Source: CAD feature listing. Evaluate the final solid. Frame: model axes, mm. Face numbers are marked on the shaded views. A direction names the side the tool comes from. Give positions to 0.01 mm unless a question says otherwise; leave off trailing zeros. Order: outer loops, then holes, each group sorted by start corner. A loop starts at its lowest first (then second) coordinate and runs counter-clockwise, first axis right, second up.
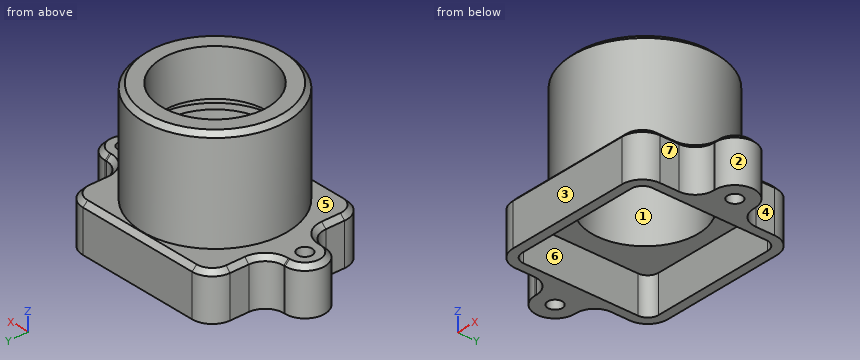
Autodesk Inventor part; units mm, degrees
ref_plane "YZ Plane" through (0, 0, 0) normal (1, 0, 0) x (0, 1, 0)
ref_plane "XZ Plane" through (0, 0, 0) normal (0, 1, 0) x (-1, 0, 0)
ref_plane "XY Plane" through (0, 0, 0) normal (0, 0, 1) x (1, 0, 0)
sketch "Boceto1" plane through (0, 0, 0) normal (0, 0, 1) x (1, 0, 0)
  line L0 (-6.67, 7.35) -> (6.67, 7.35) construction
  line L1 (7.85, 6.17) -> (7.85, -6.17) construction
  line L2 (6.67, -7.35) -> (-6.67, -7.35) construction
  line L3 (-7.85, -6.17) -> (-7.85, 6.17) construction
  line L4 (-7.85, 7.35) -> (7.85, -7.35) construction
  line L5 (7.85, 7.35) -> (-7.85, -7.35) construction
  arc A0 (-7.85, -6.17) -> (-6.67, -7.35) centre (-6.67, -6.17) ccw construction
  arc A1 (-6.67, 7.35) -> (-7.85, 6.17) centre (-6.67, 6.17) ccw construction
  arc A2 (7.85, 6.17) -> (6.67, 7.35) centre (6.67, 6.17) ccw construction
  arc A3 (6.67, -7.35) -> (7.85, -6.17) centre (6.67, -6.17) ccw construction
  line L6 (-6.67, -8.35) -> (6.67, -8.35)
  arc A4 (6.67, -8.35) -> (8.85, -6.17) centre (6.67, -6.17) ccw
  line L7 (8.85, -6.17) -> (8.85, 6.17)
  arc A5 (8.85, 6.17) -> (6.67, 8.35) centre (6.67, 6.17) ccw
  line L8 (6.67, 8.35) -> (-6.67, 8.35)
  arc A6 (-6.67, 8.35) -> (-8.85, 6.17) centre (-6.67, 6.17) ccw
  line L9 (-8.85, 6.17) -> (-8.85, -6.17)
  arc A7 (-8.85, -6.17) -> (-6.67, -8.35) centre (-6.67, -6.17) ccw
  circle A8 centre (-11, 0) radius 0.8
  circle A9 centre (11, 0) radius 0.8
  arc A10 (11, -2.15) -> (11, 2.15) centre (11, 0) ccw
  arc A11 (-11, 2.15) -> (-11, -2.15) centre (-11, 0) ccw
  line L10 (-11, 2.15) -> (-8.85, 2.15)
  line L11 (-11, -2.15) -> (-8.85, -2.15)
  line L12 (11, 2.15) -> (8.85, 2.15)
  line L13 (11, -2.15) -> (8.85, -2.15)
  point P0 (0, 0)
  point P1 (0, 0)
  point P2 (0, 0)
  dimension "d0" = 15.7
  dimension "d1" = 14.7
  dimension "d2" = 1.18
  dimension "d3" = 2.18
  dimension "d9" = 1.6
  dimension "d10" = 1.6
  dimension "d11" = 22
  dimension "d12" = 11
  dimension "d13" = 4.3
  dimension "d14" = 4.3
extrude "Extrusión1" add sketch "Boceto1" along normal blind 5 contours A7 L9 A6 L8 A5 L7 A4 L6 | L11 A11 L10 L9 | L7 L12 A10 L13 | A8 | A9
sketch "Boceto3" plane through (0, 0, 5) normal (0, 0, 1) x (1, 0, 0)
  circle A0 centre (0, 0) radius 7.8
  dimension "d15" = 15.6
extrude "Extrusión3" add sketch "Boceto3" along normal blind 11
sketch "Boceto4" plane through (0, 0, 0) normal (0, 0, -1) x (-1, 0, 0)
  line L0 (-6.67, 7.35) -> (6.67, 7.35)
  line L1 (7.85, 6.17) -> (7.85, -6.17)
  line L2 (6.67, -7.35) -> (-6.67, -7.35)
  line L3 (-7.85, -6.17) -> (-7.85, 6.17)
  line L4 (-7.85, 7.35) -> (7.85, -7.35) construction
  line L5 (7.85, 7.35) -> (-7.85, -7.35) construction
  arc A0 (-6.67, 7.35) -> (-7.85, 6.17) centre (-6.67, 6.17) ccw
  arc A1 (-7.85, -6.17) -> (-6.67, -7.35) centre (-6.67, -6.17) ccw
  arc A2 (6.67, -7.35) -> (7.85, -6.17) centre (6.67, -6.17) ccw
  arc A3 (7.85, 6.17) -> (6.67, 7.35) centre (6.67, 6.17) ccw
  point P0 (0, 0)
  dimension "d18" = 15.7
  dimension "d19" = 14.7
  dimension "d20" = 1.18
extrude "Extrusión4" cut sketch "Boceto4" against normal blind 4
sketch "Boceto5" plane through (0, 0, 16) normal (0, 0, 1) x (1, 0, 0)
  point P0 (0, 0)
hole "Agujero1" at (0, 0, 16) direction (0, 0, -1) diameter 11.459 end through all
sketch "Boceto6" plane through (0, 0, 5) normal (0, 0, 1) x (1, 0, 0)
  arc A0 (-11, 2.15) -> (-11, -2.15) centre (-11, 0) ccw construction
  arc A1 (11, -2.15) -> (11, 2.15) centre (11, 0) ccw construction
  point P0 (0, 0)
hole "Agujero2" at (-11, 0, 5) at (11, 0, 5) direction (0, 0, -1) diameter 1.567 end through all
chamfer "Chaflán1" distance 0.5 angle 45 1 edges at (-7.8, 0, 16)
fillet "Empalme1" radius 2 4 edges at (8.85, 2.15, 2.5) (8.85, -2.15, 2.5) (-8.85, 2.15, 2.5) (-8.85, -2.15, 2.5)
chamfer "Chaflán3" distance 0.5 angle 45 16 edges at (10.925, 2.15, 5) (13.15, 0, 5) (10.925, -2.15, 5) (8.85, -5.16, 5) (8.2115, -7.7115, 5) (0, -8.35, 5) (-8.2115, -7.7115, 5) (-8.85, -5.16, 5) (-10.925, -2.15, 5) (-13.15, 0, 5) (-10.925, 2.15, 5) (-8.85, 5.16, 5) (-8.2115, 7.7115, 5) (0, 8.35, 5) (8.2115, 7.7115, 5) (8.85, 5.16, 5)
sketch "Boceto9" plane through (0, 0, 0) normal (1, 0, 0) x (0, 1, 0)
  line L0 (-7.3, 16) -> (7.3, 16) construction
  line L1 (-7.8, 5) -> (7.8, 5) construction
  line L2 (-5.7295, 16) -> (5.7295, 16) construction
  line L3 (0, 16) -> (0, 5) construction
  arc A0 (6.25, 10) -> (6.25, 11) centre (6.25, 10.5) ccw
  line L4 (5.7295, 4) -> (5.7295, 16) construction
  line L5 (6.25, 11) -> (5.7295, 11)
  line L6 (6.25, 10) -> (5.7295, 10)
  line L7 (5.7295, 10) -> (5.7295, 11)
  line L8 (6.25, 10) -> (6.75, 10)
  line L9 (6.75, 10) -> (6.75, 11)
  line L10 (6.75, 11) -> (6.25, 11)
  point P0 (0, 0)
  dimension "d55" = 1
  dimension "d57" = 11.5
  dimension "d58" = 5.5
revolve "Revolución1" cut sketch "Boceto9" angle 360 about axis through (0, 0, 16) along (0, 0, -1)
properties part number "3d_DAA - M12 Lens Mount" material "Aluminium 6061-T6"
1) Material intervals for L1, parallel to X at y = 0, z = 1.3; L2, parallel to Z at x = -6, y = 1.5; L3, parallel to Y at x = 0, z = 13.55, sorted ascending.
Report:
L1: x = -13.15 to -11.78, -10.22 to -7.85, 7.85 to 10.22, 11.78 to 13.15
L2: z = 4 to 10, 11 to 16
L3: y = -7.8 to -5.73, 5.73 to 7.8
2) Section query B-B, the plane z = 15. Return the cut outline in (x, y), and give its area (3 significant figures).
Report:
outline: circle Ø15.6 at (0, 0); hole circle Ø11.46 at (0, 0)
area: 88.0 mm2
3) Section query A-A, the plane z = 3.5. Count the separate pieces of the cut face and the enclosed holes in it, and give its area (3 significant figures).
Report:
separate pieces: 1
enclosed holes: 3
area: 94.5 mm2
4) Draft query along X for the marked faces 1, 2 and 3. Return one class per face: +X half, -X half, draft (parallel to the pull), parting line (faces both ways), or undercut.
Report:
face 1: undercut
face 2: +X half
face 3: draft
5) Reachability of the marked faces 4, 5, 6 and 7 from +Z, -Z, +X, -X, +Y, -Y: full face, straight path, thin tool, end or side. Return the list, or none.
Report:
face 4: +Z, -Z, +X, +Y
face 5: +Z
face 6: -Z
face 7: +Z, -Z, +X, -Y
6) Pin query (flat end, axial travel): pin 1 (6 mm diameter, centred on y = 1, z = 10.5, fed in from -X); pin 2 (1 mm diameter, centred on y = -5.5, z = 2, fed in from -X); pin 3 (2 mm diameter, centred on x = -11, y = 0, fed in from +Z). Return the tip coordinate at first contact, or that it passes through.
Report:
pin 1: stops at x = -7.8
pin 2: stops at x = -8.85
pin 3: stops at z = 5
